```python
from build123d import *

# Parameters (mm, degrees)
F3_D     = 8.5
F3_DEPTH = 25
F3_TIP   = 2.5536576309
F5_D     = 11
F5_DEPTH = 30
F5_TIP   = 3.3047334047


with BuildPart() as f1:
    # F0 (on Front) → F1 (revolve)
    with BuildSketch(Plane.XZ):
        Polygon((0, 53), (0, 0), (8.5, 0), (8.5, 50), (15, 50), (15, 53), align=None)
    revolve(axis=Axis((0, 0, 35.806838423), (0, 0, 1)))

    # F3
    with Locations(Plane.XY.offset(53)):
        with Locations((0, 0)):
            Hole(F3_D / 2, depth=F3_DEPTH)
            with Locations((0, 0, -(F3_DEPTH + F3_TIP / 2))):  # 118° drill point
                Cone(0, F3_D / 2, F3_TIP, mode=Mode.SUBTRACT)

    # F5
    with Locations(Plane(origin=(0, 0, 0), x_dir=(1, 0, 0), z_dir=(0, 0, -1))):
        with Locations((0, 0)):
            Hole(F5_D / 2, depth=F5_DEPTH)
            with Locations((0, 0, -(F5_DEPTH + F5_TIP / 2))):  # 118° drill point
                Cone(0, F5_D / 2, F5_TIP, mode=Mode.SUBTRACT)


solid = f1.part
```
Geometry: final body of the model. Coordinates: model frame, mm. A direction names the side the tool comes from. Round coordinates to 2 decimals unless told otherwise and drop trailing zeros. Order: outer loops, then holes, each group sorted by start corner. A loop starts at its lowest first (then second) coordinate and runs counter-clockwise, first axis right, second up. Notation, with made-up numbers: (66, -21) -> (116, -21) arc R17 cw to (116, 10) -> close; hole circle Ø9 at (10.25, 51.25). An arc over 180 degrees is marked (long way). Use CSV: the item, a comma, the result in double quotes. Start each with the question number.
1) Set-up query: faces 4 (the face through (4.57, 7.167, 25.35)), 5 (the face through (3.12, -3.12, 53)). Return all of +Z, -Z, +X, -X, +Y, -Y with unobstructed straight access to the full face (end or side cutting, diameter ignored); none if empty.
2) First-contact query: pin 1 Ø3 at (x, z) = (6.5, 36.5) entering from +Y; pin 2 Ø3 at (y, z) = (1, 30) entering from +X; pin 3 Ø12 at (x, z) = (-2.5, 36) entering from -Y; pin 4 Ø5 at (x, y) = (0, 0) entering from +Z. Flat tips, straight axial feed; report the tip coordinate or a pass-through.
3) Draft query along Y for faces 1 (the face through (1.19, 5.37, 15.21)), 2 (the face through (-6.5, -6.5, 50)), 3 (the face through (-14.985, 0.66, 51.521)). Return one class per face: +Y half, -Y half, draft (parallel to the pull), parting line (faces both ways), or undercut.
4) Material intervals for line 1 along Y through (x, z) = (0.25, 27); line 2 along Z through (x, y) = (10, -6.25); line 3 along X through (y, z) = (1.25, 6.5), sorted ascending. Write a range as from..to.
5) Section C-C (z = 11.5). Return the cut outline in (x, y).
6) Section D-D (y = 12). Return the cut outline in (x, z), and give its area (3 significant figures).
7) Section A-A (x = 0). Return the cut outline in (y, z).
Returned:
1,face 4,"-Z"
1,face 5,"+Z, +X, -X, +Y, -Y"
2,pin 1,"stops at y = 6.87"
2,pin 2,"stops at x = 8.5"
2,pin 3,"stops at y = -8.5"
2,pin 4,"passes through"
3,face 1,"undercut"
3,face 2,"draft"
3,face 3,"parting line"
4,line 1,"y = -8.5..-5.49, 5.49..8.5"
4,line 2,"z = 50..53"
4,line 3,"x = -8.41..-5.36, 5.36..8.41"
5,outline,"circle Ø17 at (0, 0); hole circle Ø11 at (0, 0)"
6,outline,"(-9, 50) -> (9, 50) -> (9, 53) -> (-9, 53) -> close"
6,area,"54.0 mm²"
7,outline,"(-15, 50) -> (-8.5, 50) -> (-8.5, 0) -> (-5.5, 0) -> (-5.5, 30) -> (-4.25, 30.75) -> (-4.25, 53) -> (-15, 53) -> close; (4.25, 30.75) -> (5.5, 30) -> (5.5, 0) -> (8.5, 0) -> (8.5, 50) -> (15, 50) -> (15, 53) -> (4.25, 53) -> close"
